Source: CAD feature listing. Evaluate the final solid. Frame: model axes, mm. A direction names the side the tool comes from. Give positions to 0.01 mm unless a question says otherwise; leave off trailing zeros. Order: outer loops, then holes, each group sorted by start corner. A loop starts at its lowest first (then second) coordinate and runs counter-clockwise, first axis right, second up. Notation, with made-up numbers: M 23.5,12.25 L 35.5,12.25 A36 ccw 35.5,50.25 Z; hole C -11.5,2 d2. An arc over 180 degrees is marked long. Use CSV: the item, a comma, the result in double quotes. Start each with the question number.
Item 1: Pull-direction query (X, two-part tool) for faces 1 (the face through (19, -13, 15)), 2 (the face through (32.6, -32.82, 7.4)), 3 (the face through (-4.434, 31.516, 7.395)); classes: +X half, -X half, draft (parallel to the pull), parting line (faces both ways), or undercut.
Item 2: Section query D-D on x = -20. Return loops of the section in (y, z), and give its area (3 significant figures).
Item 3: Access query for faces 4 (the face through (12, 3, 0)), 5 (the face through (-17.644, -14.109, 7.395)), 6 (the face through (5.43, 66.016, 31.014)), 7 (the face through (7.696, 2.398, 7.395)). Directions: +Z, -Z, +X, -X, +Y, -Y. A direction counts if a zero-diameter tool reaches every point of the face in a straight line with its end or side. Return the directions, or none.
Item 4: Section query B-B on x = 7. Return loops of the section in (y, z), and give its area (3 significant figures).
Item 5: First-contact query: pin 1 (10 mm diameter, centred on x = -8, z = 14.5, fed in from -Y); pin 2 (2 mm diameter, centred on x = 33, y = 45, fed in from +Z); pin 3 (12 mm diameter, centred on x = -21.5, z = 13, fed in from +Y). Flat tips, straight axial feed; report the tip coordinate or a pass-through.
Item 6: Section query C-C on y = 16. Return loops of the section in (x, z).
Item 7: Ray query, probe 1 along X at (y, z) = (-23, 4.5); probe 2 along Y at (x, z) = (0, 7); probe 3 along Z at (x, y) = (10, -47). Return the intervals inside material, ascending. Write a range as from..to.
from build123d import *

# Parameters (mm, degrees)
EXTRUDE_1_DEPTH     = 15
SKETCH_6_R          = 3.5
CUT_EXTRUDE_2_DEPTH = 15
SKETCH_9_R          = 15
SKETCH_9_R_2        = 3.5
EXTRUDE_2_DEPTH     = 17
SKETCH_10_R         = 10.1
CUT_EXTRUDE_5_DEPTH = 2


with BuildPart() as part:
    # ｽｹｯﾁ1 → ﾎﾞｽ - 押し出し1 (new body)
    with BuildSketch(Plane.XY):
        with BuildLine():
            Line((10.546944731, 68.165925034), (9.641814145, 68.990666647))
            ThreePointArc((9.641814145, 68.990666647), (-9.131421435, 69.400300104), (-13.594616806, 51.160726074))
            Line((-13.594616806, 51.160726074), (4.986432096, 11.313538113))
            ThreePointArc((4.986432096, 11.313538113), (5.221931994, 9.524738795), (4.388829079, 7.924362985))
            Line((4.388829079, 7.924362985), (-40.303464689, -36.767930783))
            ThreePointArc((-40.303464689, -36.767930783), (-41.182112782, -38.903012739), (-40.283913759, -41.029943849))
            ThreePointArc((-40.283913759, -41.029943849), (41.397896806, -39.905690573), (39.524106652, 41.762363359))
            Line((39.524106652, 41.762363359), (37.916838192, 43.226882625))
            Line((37.916838192, 43.226882625), (10.546944731, 68.165925034))
        make_face()
        with BuildLine():
            ThreePointArc((5.093338956, 1.55780505), (7.735603832, 2.390907965), (9.933582661, 0.704339492))
            Line((9.933582661, 0.704339492), (27.046217634, -35.993824637))
            ThreePointArc((27.046217634, -35.993824637), (27.212084573, -38.085077821), (25.967336583, -39.773702754))
            ThreePointArc((25.967336583, -39.773702754), (-1.972837213, -47.459012983), (-29.17877254, -37.481318454))
            ThreePointArc((-29.17877254, -37.481318454), (-30.330146685, -35.299826939), (-29.457223039, -32.992756945))
            Line((-29.457223039, -32.992756945), (5.093338956, 1.55780505))
        make_face(mode=Mode.SUBTRACT)
        with BuildLine():
            ThreePointArc((35.231836325, -31.858557864), (32.560090836, -32.813013733), (30.287744354, -31.114293205))
            Line((30.287744354, -31.114293205), (-2.054746852, 38.244403012))
            ThreePointArc((-2.054746852, 38.244403012), (-1.895310582, 41.077194163), (0.553480425, 42.510214831))
            ThreePointArc((0.553480425, 42.510214831), (5.039223996, 43.371793408), (9.057681155, 45.543478261))
            ThreePointArc((9.057681155, 45.543478261), (10.270904088, 46.091905397), (11.601973614, 46.061309233))
            ThreePointArc((11.601973614, 46.061309233), (45.455779175, 13.784851815), (35.231836325, -31.858557864))
        make_face(mode=Mode.SUBTRACT)
    extrude(amount=EXTRUDE_1_DEPTH)

    # ｽｹｯﾁ6 → ｶｯﾄ - 押し出し2 (cut)
    with BuildSketch(Plane.XY.offset(15)):
        with Locations((0, 57.5)):
            Circle(SKETCH_6_R)
    extrude(amount=-CUT_EXTRUDE_2_DEPTH, mode=Mode.SUBTRACT)

    # ｽｹｯﾁ9 → ﾎﾞｽ - 押し出し2 (add)
    with BuildSketch(Plane.XY.offset(15)):
        with Locations(Location((0, 57.5, 0), (0, 0, 205))):
            Circle(SKETCH_9_R)
        with Locations((0, 57.5)):
            Circle(SKETCH_9_R_2, mode=Mode.SUBTRACT)
    extrude(amount=EXTRUDE_2_DEPTH)

    # ｽｹｯﾁ10 → ｶｯﾄ - 押し出し5 (cut)
    with BuildSketch(Plane.XY.offset(32)):
        with Locations((0, 57.5)):
            Circle(SKETCH_10_R)
    extrude(amount=-CUT_EXTRUDE_5_DEPTH, mode=Mode.SUBTRACT)


solid = part.part
Verdict:
1,face 1,"draft"
1,face 2,"undercut"
1,face 3,"-X half"
2,outline,"M -53.91,0 L -43.08,0 L -43.08,15 L -53.91,15 Z; M -23.54,0 L -16.46,0 L -16.46,15 L -23.54,15 Z"
2,area,"268 mm2"
3,face 4,"-Z, +X, -X, +Y, -Y"
3,face 5,"+Z, -Z, -X"
3,face 6,"+Z"
3,face 7,"+Z, -Z"
4,outline,"M -57.07,0 L -46.98,0 L -46.98,15 L -57.07,15 Z; M 2.43,0 L 18.83,0 L 18.83,15 L 2.43,15 Z; M 44.23,0 L 70.77,0 L 70.77,32 L 64.78,32 L 64.78,30 L 50.22,30 L 50.22,32 L 44.23,32 Z"
4,area,"1,220 mm2"
5,pin 1,"y = -57.42"
5,pin 2,"z = 15"
5,pin 3,"y = -11.96"
6,outline,"M 2.8,0 L 8.32,0 L 8.32,15 L 2.8,15 Z; M 44.72,0 L 55.23,0 L 55.23,15 L 44.72,15 Z"
7,probe 1,"-26.54..-19.46, 20.99..26.5, 41.56..52.7"
7,probe 2,"-57.5..-47.5, -3.54..3.54, 22.01..33.84, 42.44..54, 61..72.5"
7,probe 3,"0..15"
